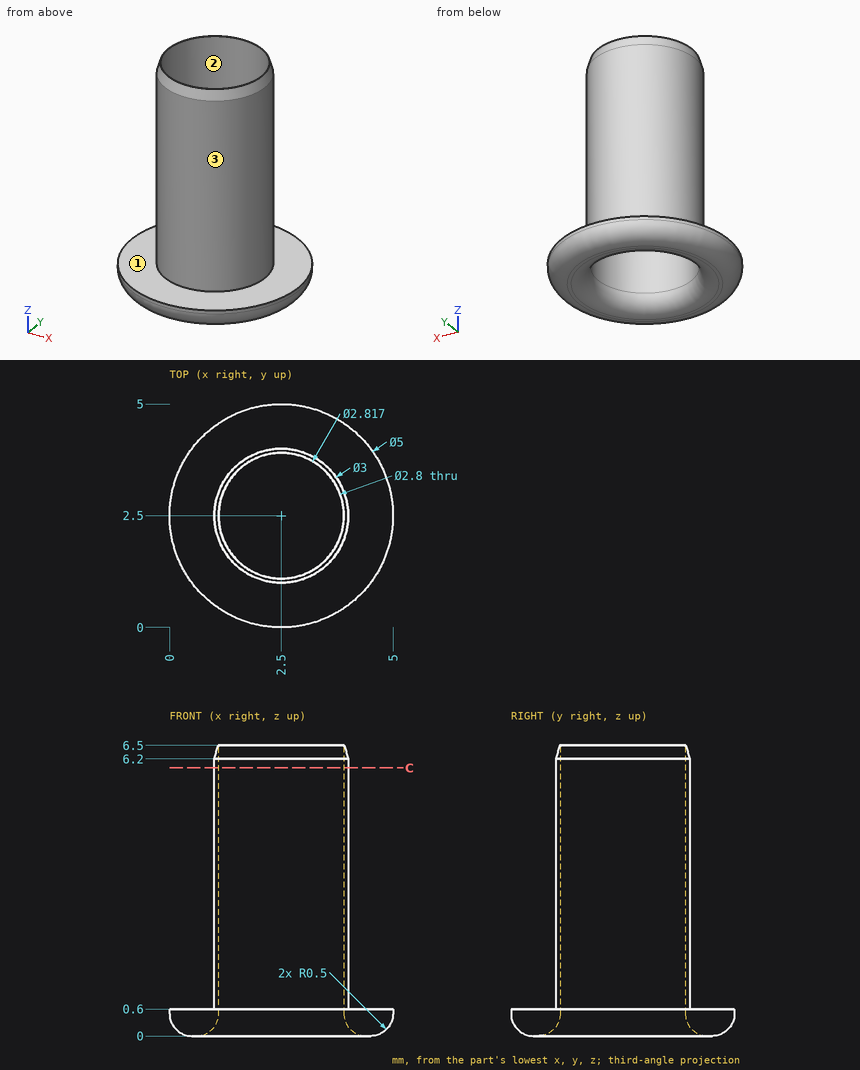
Here's the drawing with two shaded views (mm, measured from the low corner). I have some questions. Coordinates: 2 decimals unless noted, no trailing zeros. Write each loop counter-clockwise with the first axis right and the second up, starting at its lowest first coordinate (ties: lowest second). Pieces come first, ordered by that corner, then holes. Notation, with made-up numbers: M -35,59 L -14,59 A23 cw -14,83 Z; hole C 79.5,-19 d7. An arc over 180 degrees is marked long. Answer as CSV lines item,"result". Start each with the question number.
1) We'd pull the mould along Y, two halves only. Please class the marked faces 1, 2 and 3: +Y half, -Y half, draft (parallel to the pull), parting line (faces both ways), or undercut.
2) For P1, Ø1, axis at x = 1, z = 1.5, coming from the +Y side, with a flat end and sliding along its axis, tell me the tip position at first contact or that it passes through.
3) Please list where these lines run through material, in increasing order: line 1 (Z direction, x = 4, y = 1.35); line 2 (X direction, y = 3.05, z = 0.5); line 3 (Z direction, x = 4.1, y = 2.6). Write a range as from..to.
4) I want a section at C-C, the plane z = 6. Please give me the cut outline in (x, y).
Data:
1,face 1,"draft"
1,face 2,"undercut"
1,face 3,"parting line"
2,P1,"stops at y = 3.62"
3,line 1,"z = 0..0.6"
3,line 2,"x = 0.06..1.21, 3.79..4.94"
3,line 3,"z = 0.1..0.6"
4,outline,"C 2.5,2.5 d3; hole C 2.5,2.5 d2.8"
